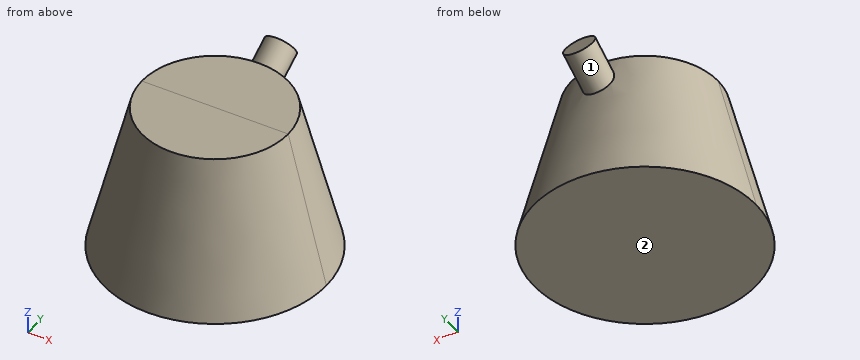
from build123d import *

# Parameters (mm, degrees)
F1_ANGLE = 180
F4_R     = 6.68337
F5_DEPTH = 40


with BuildPart() as f1:
    # F0 (on Front) → F1 (revolve)
    with BuildSketch(Plane.XZ):
        Polygon((0, 64.147353), (0, 0), (47.980133, 0), (31.552151, 64.147353), align=None)
    revolve(axis=Axis((0, 0, 32.073677), (0, 0, -1)), revolution_arc=F1_ANGLE)

    # F3: F1 across plane


with BuildPart() as f1_1:
    add(f1.part)
    add(f1.part.mirror(Plane.XZ))

    # F4 (on face) → F5 (join)
    with BuildSketch(Plane(origin=(0, 27.776619, 16.036838), x_dir=(-1, 0, 0), z_dir=(0, 0.866025, 0.5))):
        with Locations((0, 29.759701)):
            Circle(F4_R)
    extrude(amount=F5_DEPTH)


solid = f1_1.part
Design review of the part built by this model. Coordinates are the model's own, in mm. Face numbers are marked on the shaded views. Give positions to 0.01 mm unless a question says otherwise; leave off trailing zeros. Write each loop counter-clockwise with the first axis right and the second up, starting at its lowest first coordinate (ties: lowest second). Pieces come first, ordered by that corner, then holes. Notation, with made-up numbers: M 19,75 L 48,75 A6 cw 48,83 Z; hole C 8.5,84.5 d10. An arc over 180 degrees is marked long. Answer as a JSON object with one key per item and string values. Group by question number.
1) We need section B-B (z = 31.5). Give the boundary of the cut face in (x, y).
2) We need section C-C (z = 24). Give the boundary of the cut face in (x, y).
3) We need section A-A (x = 0). Give the boundary of the cut face in (y, z).
4) Clearance check with flat-ended pins moving along their axes: pin 1 Ø1.5 at (y, z) = (33.5, 10.5) entering from +X; pin 2 Ø3 at (x, z) = (-8, 10) entering from -Y; pin 3 Ø1.5 at (y, z) = (31.5, 9) entering from -X. State where each tip first meets the part, or that it passes through.
5) For line 1 along Z through (x, y) = (6, 9); line 2 along X through (y, z) = (25, 10); line 3 along X through (y, z) = (-19, 36.5), list the stretches that pass through material, from the lowest coordinate up.
6) Mouldability with a two-part tool opening along Z and no side actions: class the marked faces 1 and 2 as released by +Z, released by -Z, zero draft, split by the parting line, or undercut.
Answer key:
{
 "1": {"outline": "C 0,0 d79.83"},
 "2": {"outline": "C 0,0 d83.67"},
 "3": {"outline": "M -47.98,0 L 47.98,0 L 35.85,47.35 L 50.88,56.02 L 44.2,67.6 L 32.41,60.79 L 31.55,64.15 L -31.55,64.15 Z"},
 "4": {"pin 1": "stops at x = 31.33", "pin 2": "stops at y = -45.17", "pin 3": "stops at x = -33.82"},
 "5": {"line 1": "z = 0 to 64.15", "line 2": "x = -37.92 to 37.92", "line 3": "x = -33.64 to 33.64"},
 "6": {"face 1": "undercut", "face 2": "released by -Z"}
}
